The model under review builds one solid part; all positions refer to its coordinate system, in mm. A direction names the side the tool comes from. Coordinates: 2 decimals unless noted, no trailing zeros. Write each loop counter-clockwise with the first axis right and the second up, starting at its lowest first coordinate (ties: lowest second). Pieces come first, ordered by that corner, then holes.
```python
from build123d import *

# Parameters (mm, degrees)
SKETCH1_R             = 1.6
BOSS_EXTRUDE1_DEPTH   = 8
SKETCH2_W             = 9
SKETCH2_H             = 8.199711987
CUT_EXTRUDE1_DEPTH    = 8
BOSS_EXTRUDE2_DEPTH   = 6
SKETCH4_R             = 1.6
BOSS_EXTRUDE3_DEPTH   = 8
SKETCH5_W             = 24.599859369
SKETCH5_H             = 11.841190876
CUT_EXTRUDE2_DEPTH    = 10
SKETCH6_W             = 21
SKETCH6_H             = 36
SKETCH6_R             = 1.6
SKETCH6_W_2           = 9
SKETCH6_H_2           = 24
BOSS_EXTRUDE4_DEPTH   = 8
LPATTERN1_OUTLINE_R   = 1.6
LPATTERN1_DEPTH       = 8
LPATTERN1_2_OUTLINE_W = 9
LPATTERN1_2_OUTLINE_H = 6
LPATTERN1_2_DEPTH     = 2
LPATTERN1_START       = -33
LPATTERN1_3_DEPTH     = 6
FILLET1_R             = 2.5
CHAMFER1_SIZE         = 1


with BuildPart() as part:
    # Sketch1 → Boss-Extrude1 (new body)
    with BuildSketch(Plane.XY):
        with BuildLine():
            Line((-0.5, 3), (15.5, 3))
            ThreePointArc((15.5, 3), (17.267766953, 2.267766953), (18, 0.5))
            Line((18, 0.5), (18, -0.5))
            ThreePointArc((18, -0.5), (17.267766953, -2.267766953), (15.5, -3))
            Line((15.5, -3), (-0.5, -3))
            ThreePointArc((-0.5, -3), (-2.267766953, -2.267766953), (-3, -0.5))
            Line((-3, -0.5), (-3, 0.5))
            ThreePointArc((-3, 0.5), (-2.267766953, 2.267766953), (-0.5, 3))
        make_face()
        Circle(SKETCH1_R, mode=Mode.SUBTRACT)
        with Locations((15, 0)):
            Circle(SKETCH1_R, mode=Mode.SUBTRACT)
    boss_extrude1 = extrude(amount=BOSS_EXTRUDE1_DEPTH)

    # Sketch2 → Cut-Extrude1 (cut)
    with BuildSketch(Plane.XZ.offset(3)):
        with Locations((7.5, 6.099855994)):
            Rectangle(SKETCH2_W, SKETCH2_H)
    cut_extrude1 = extrude(amount=-CUT_EXTRUDE1_DEPTH, mode=Mode.SUBTRACT)

    # Sketch3 → Boss-Extrude2 (add)
    with BuildSketch(Plane.XZ.offset(3)):
        Polygon((3.257359313, 2), (7.5, 6.242640687), (11.742640687, 2), align=None)
    boss_extrude2 = extrude(amount=-BOSS_EXTRUDE2_DEPTH)

    # Sketch4 → Boss-Extrude3 (add)
    # profile 1 of 2: a face of its own
    with BuildSketch(Plane(origin=(0, 0, 0), x_dir=(-1, 0, 0), z_dir=(0, 0, -1))):
        with BuildLine():
            Line((15.5, 3), (0.5, 3))
            ThreePointArc((0.5, 3), (2.267766953, 2.267766953), (3, 0.5))
            Line((3, 0.5), (3, -0.5))
            ThreePointArc((3, -0.5), (2.267766953, -2.267766953), (0.5, -3))
            Line((0.5, -3), (15.5, -3))
            ThreePointArc((15.5, -3), (17.267766953, -2.267766953), (18, -0.5))
            Line((18, -0.5), (18, 0.5))
            ThreePointArc((18, 0.5), (17.267766953, 2.267766953), (15.5, 3))
        make_face()
        with Locations((7.5, 0)):
            Circle(SKETCH4_R, mode=Mode.SUBTRACT)
        with Locations((15, 0)):
            Circle(SKETCH4_R, mode=Mode.SUBTRACT)
    # profile 2 of 2: a face of its own
    with BuildSketch(Plane(origin=(0, 0, 0), x_dir=(-1, 0, 0), z_dir=(0, 0, -1))):
        with BuildLine():
            ThreePointArc((-18, 0.5), (-17.267766953, 2.267766953), (-15.5, 3))
            Line((-15.5, 3), (-30.5, 3))
            ThreePointArc((-30.5, 3), (-32.267766953, 2.267766953), (-33, 0.5))
            Line((-33, 0.5), (-33, -0.5))
            ThreePointArc((-33, -0.5), (-32.267766953, -2.267766953), (-30.5, -3))
            Line((-30.5, -3), (-15.5, -3))
            ThreePointArc((-15.5, -3), (-17.267766953, -2.267766953), (-18, -0.5))
            Line((-18, -0.5), (-18, 0.5))
        make_face()
        with Locations((-30, 0)):
            Circle(SKETCH4_R, mode=Mode.SUBTRACT)
        with Locations((-22.5, 0)):
            Circle(SKETCH4_R, mode=Mode.SUBTRACT)
    boss_extrude3 = extrude(amount=-BOSS_EXTRUDE3_DEPTH)

    # Sketch5 → Cut-Extrude2 (cut)
    with BuildSketch(Plane.XY.offset(8)):
        with Locations((-9.299929685, -2.920595438)):
            Rectangle(SKETCH5_W, SKETCH5_H)
    extrude(amount=-CUT_EXTRUDE2_DEPTH, mode=Mode.SUBTRACT)

    # Sketch6 → Boss-Extrude4 (add)
    with BuildSketch(Plane(origin=(0, 0, 0), x_dir=(-1, 0, 0), z_dir=(0, 0, -1))):
        with Locations((7.5, -15)):
            Rectangle(SKETCH6_W, SKETCH6_H)
        Circle(SKETCH6_R, mode=Mode.SUBTRACT)
        with Locations((7.5, 0)):
            Circle(SKETCH6_R, mode=Mode.SUBTRACT)
        with Locations((15, 0)):
            Circle(SKETCH6_R, mode=Mode.SUBTRACT)
        with Locations((0, -7.5)):
            Circle(SKETCH6_R, mode=Mode.SUBTRACT)
        with Locations((0, -15)):
            Circle(SKETCH6_R, mode=Mode.SUBTRACT)
        with Locations((0, -22.5)):
            Circle(SKETCH6_R, mode=Mode.SUBTRACT)
        with Locations((0, -30)):
            Circle(SKETCH6_R, mode=Mode.SUBTRACT)
        with Locations(Location((15, -30, 0), (0, 0, 180))):
            Circle(SKETCH6_R, mode=Mode.SUBTRACT)
        with Locations(Location((7.5, -30, 0), (0, 0, 180))):
            Circle(SKETCH6_R, mode=Mode.SUBTRACT)
        with Locations(Location((15, -22.5, 0), (0, 0, 180))):
            Circle(SKETCH6_R, mode=Mode.SUBTRACT)
        with Locations(Location((15, -15, 0), (0, 0, 180))):
            Circle(SKETCH6_R, mode=Mode.SUBTRACT)
        with Locations(Location((15, -7.5, 0), (0, 0, 180))):
            Circle(SKETCH6_R, mode=Mode.SUBTRACT)
        with Locations((7.5, -15)):
            Rectangle(SKETCH6_W_2, SKETCH6_H_2, mode=Mode.SUBTRACT)
    boss_extrude4 = extrude(amount=-BOSS_EXTRUDE4_DEPTH)



with BuildPart() as body_2:
    # LPattern1: read off the stored shape, not the designer's step
    # LPattern1 outline → LPattern1 (new body)
    with BuildSketch(Plane.XY):
        with BuildLine():
            Line((12, -27), (12, -33))
            Line((12, -33), (30.5, -33))
            ThreePointArc((30.5, -33), (32.267766953, -32.267766953), (33, -30.5))
            Line((33, -30.5), (33, -29.5))
            ThreePointArc((33, -29.5), (32.267766953, -27.732233047), (30.5, -27))
            Line((30.5, -27), (12, -27))
        make_face()
        with Locations((15, -30)):
            Circle(LPATTERN1_OUTLINE_R, mode=Mode.SUBTRACT)
        with Locations((22.5, -30)):
            Circle(LPATTERN1_OUTLINE_R, mode=Mode.SUBTRACT)
        with Locations((30, -30)):
            Circle(LPATTERN1_OUTLINE_R, mode=Mode.SUBTRACT)
    lpattern1 = extrude(amount=LPATTERN1_DEPTH)


with BuildPart() as part_1:
    add(part.part)

    add(body_2.part)  # LPattern1 2 merges body 2
    # LPattern1 2 outline → LPattern1 2 (add)
    with BuildSketch(Plane.XY):
        with Locations((7.5, -30)):
            Rectangle(LPATTERN1_2_OUTLINE_W, LPATTERN1_2_OUTLINE_H)
    lpattern1_2 = extrude(amount=LPATTERN1_2_DEPTH)

    # LPattern1 3 outline → LPattern1 3 (add)
    with BuildSketch(Plane(origin=(0, 0, 0), x_dir=(1, 0, 0), z_dir=(0, 1, 0)).offset(LPATTERN1_START)):
        Polygon((11.742640687, -2), (3.257359313, -2), (7.5, -6.242640687), align=None)
    lpattern1_3 = extrude(amount=LPATTERN1_3_DEPTH)

    # Mirror1: Boss-Extrude1, Cut-Extrude1, Boss-Extrude2, Boss-Extrude3, Boss-Extrude4, LPattern1, LPattern1 2, LPattern1 3 across plane
    add(boss_extrude1.mirror(Plane.ZY.offset(7.5)))
    add(cut_extrude1.mirror(Plane.ZY.offset(7.5)), mode=Mode.SUBTRACT)
    add(boss_extrude2.mirror(Plane.ZY.offset(7.5)))
    add(boss_extrude3.mirror(Plane.ZY.offset(7.5)))
    add(boss_extrude4.mirror(Plane.ZY.offset(7.5)))
    add(lpattern1.mirror(Plane.ZY.offset(7.5)))
    add(lpattern1_2.mirror(Plane.ZY.offset(7.5)))
    add(lpattern1_3.mirror(Plane.ZY.offset(7.5)))

    # Fillet1
    fillet1_edges = [part_1.edges().sort_by_distance(p)[0] for p in [
        (-12, -3, 4),
        (-12, -27, 4),
        (-3, -27, 4),
        (-3, -3, 4),
    ]]
    fillet(fillet1_edges, radius=FILLET1_R)

    # Chamfer1
    chamfer1_edges = [part_1.edges().sort_by_distance(p)[0] for p in [
        (-16.6, -7.5, 8),
        (-16.6, -15, 8),
        (-16.6, -22.5, 8),
        (-9.1, -30, 8),
        (-16.6, -30, 8),
        (1.6, -30, 8),
        (1.6, -22.5, 8),
        (1.6, -15, 8),
        (1.6, -7.5, 8),
        (-13.4, 0, 8),
        (-5.9, 0, 8),
        (1.6, 0, 8),
        (1.6, 0, 0),
        (-5.9, 0, 0),
        (-13.4, 0, 0),
        (1.6, -7.5, 0),
        (1.6, -15, 0),
        (1.6, -22.5, 0),
        (1.6, -30, 0),
        (-16.6, -30, 0),
        (-9.1, -30, 0),
        (-16.6, -22.5, 0),
        (-16.6, -15, 0),
        (-16.6, -7.5, 0),
        (13.4, 0, 0),
        (13.4, 0, 8),
        (13.4, -30, 0),
        (13.4, -30, 8),
        (28.4, -30, 8),
        (20.9, -30, 8),
        (28.4, -30, 0),
        (20.9, -30, 0),
        (-28.4, 0, 8),
        (-28.4, 0, 0),
        (-46.6, 0, 0),
        (-39.1, 0, 0),
        (-46.6, 0, 8),
        (-39.1, 0, 8),
        (-28.4, -30, 8),
        (-28.4, -30, 0),
        (-43.4, -30, 0),
        (-35.9, -30, 0),
        (-43.4, -30, 8),
        (-35.9, -30, 8),
        (31.6, 0, 8),
        (24.1, 0, 8),
        (31.6, 0, 0),
        (24.1, 0, 0),
    ]]
    chamfer(chamfer1_edges, length=CHAMFER1_SIZE)


solid = part_1.part
```
Item 1: Take a section at A-A, the plane x = -4. Write out the cut boundary in (y, z), plus the area to 3 significant figures.
Solved:
outline: (-33, 0) - (-26.5, 0) - (-26.5, 8) - (-33, 8) - close; (-3.5, 0) - (3, 0) - (3, 8) - (-3.5, 8) - close
area: 104 mm2
Item 2: Mouldability with a two-part tool opening along Y and no side actions: class faces 5 (the face through (25, 1.4, 8)), 6 (the face through (-46.18, 1.08, 3.96)) as pulls with the +Y half, pulls with the -Y half, needs draft (parallel to the pull), parting line crosses it, or undercut.
Solved:
face 5: needs draft
face 6: undercut
Item 3: For pin 1 (2 mm diameter, centred on y = -26.5, z = 6, fed in from +X); pin 2 (4 mm diameter, centred on x = 0, y = -22.5, fed in from -Z); pin 3 (4 mm diameter, centred on y = -15.5, z = 3.5, fed in from -X), all flat-tipped, find the tip position at first contact; note any pin that passes through.
Solved:
pin 1: stops at x = 32
pin 2: stops at z = 0.6
pin 3: stops at x = -18
Item 4: Take a section at C-C, the plane x = -15. Count the separate pieces of the cut face and the enclosed holes in it, plus the area to 3 significant figures.
Solved:
separate pieces: 6
enclosed holes: 0
area: 150 mm2
Item 5: To check wall thickness, follow line 1 along Y through (x, z) = (0, 5.6); line 2 along Y through (x, z) = (30, 3.9); line 3 along Y through (x, z) = (-34.5, 2). State the ranges of each line that lie inside material, in increasing order.
Solved:
line 1: y = -33 to -31.6, -28.4 to -24.1, -20.9 to -16.6, -13.4 to -9.1, -5.9 to -1.6, 1.6 to 3
line 2: y = -33 to -31.6, -28.4 to -27, -3 to -1.6, 1.6 to 3
line 3: y = -33 to -27, -3 to 3
Item 6: Take a section at B-B, the plane y = -7.5. Write out the cut boundary in (x, z).
Solved:
outline: (-18, 0) - (-17.6, 0) - (-16.6, 1) - (-16.6, 7) - (-17.6, 8) - (-18, 8) - close; (-13.4, 1) - (-12.4, 0) - (-12, 0) - (-12, 8) - (-12.4, 8) - (-13.4, 7) - close; (-3, 0) - (-2.6, 0) - (-1.6, 1) - (-1.6, 7) - (-2.6, 8) - (-3, 8) - close; (1.6, 1) - (2.6, 0) - (3, 0) - (3, 8) - (2.6, 8) - (1.6, 7) - close
Item 7: Machinability: for faces 1 (the face through (-18, -15, 4)), 2 (the face through (-11.287, -26.248, 4.056)), 3 (the face through (12, -30, 5)), 4 (the face through (-47.287, -27.752, 3.944)), which of the approach directions +Z, -Z, +X, -X, +Y, -Y give a long, thin tool a straight path to every point of the face, cutting with its end or side? Answer none if there is none.
Solved:
face 1: +Z
face 2: +Z, -Z
face 3: +Z, +Y, -Y
face 4: +Z, -Z, -X
